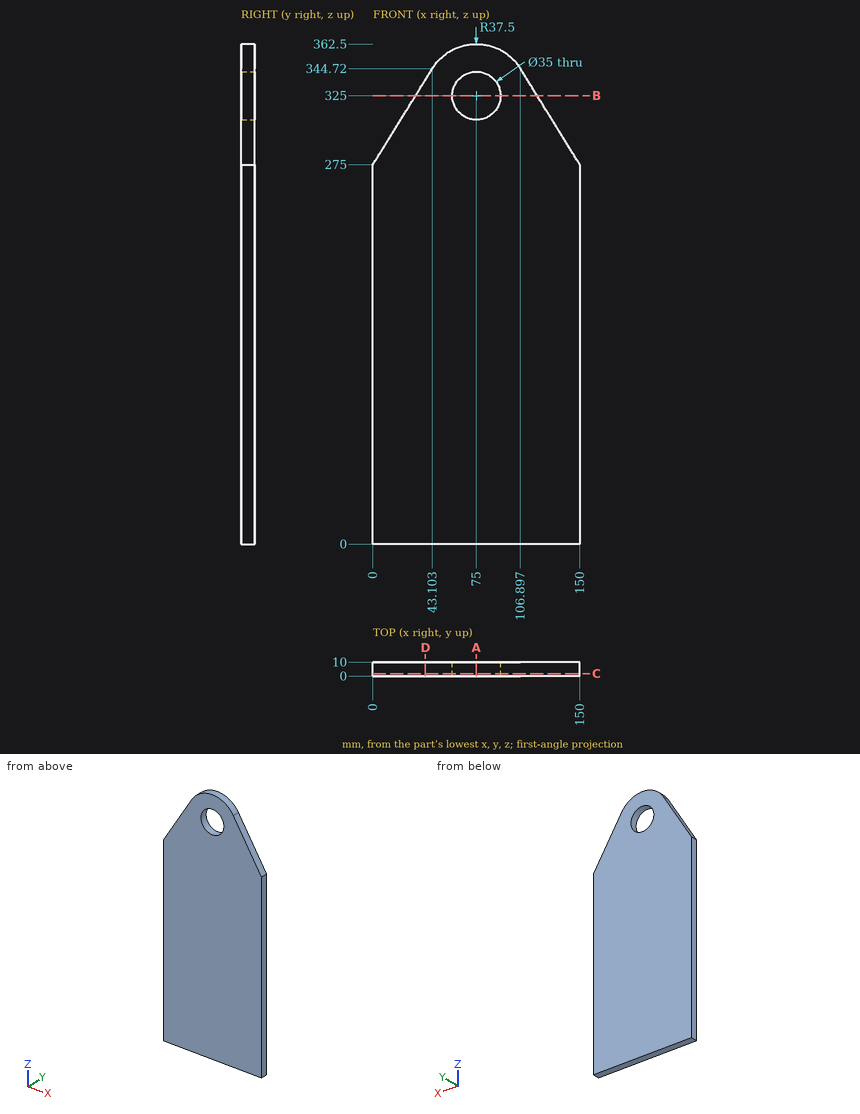
Input: dimensioned drawing with shaded views. Units: mm. Origin: part minimum x, y, z. Coordinates: 2 decimals unless noted, no trailing zeros. Order: outer loops, then holes, each group sorted by start corner. A loop starts at its lowest first (then second) coordinate and runs counter-clockwise, first axis right, second up.
1. Cut plane B-B, the plane z = 325. Return loops of the section in (x, y), plus the area to 3 significant figures.
Checked values:
outline: (30.91, 0) - (57.5, 0) - (57.5, 10) - (30.91, 10) - close; (92.5, 0) - (119.09, 0) - (119.09, 10) - (92.5, 10) - close
area: 532 mm2
2. Cut plane C-C, the plane y = 1.75. Return loops of the section in (x, z).
Checked values:
outline: (0, 0) - (150, 0) - (150, 275) - (106.9, 344.72) arc R37.5 ccw to (43.1, 344.72) - (0, 275) - close; hole circle Ø35 at (75, 325)
3. Contact query for a flat-ended pin moving along its axis: P1, Ø1, axis at x = 45.5, y = 3.5, coming from the +Z side (1 decimal). Output: stop coordinate, or through.
Checked values:
P1: stops at z = 348.8
4. Ray query, line 1 along Z through (x, y) = (75, 5); line 2 along Z through (x, y) = (63, 8.75) (1 decimal); line 3 along Z through (x, y) = (122, 6.5). Return the intervals inside material, ascending.
Checked values:
line 1: z = 0 to 307.5, 342.5 to 362.5
line 2: z = 0 to 312.3, 337.7 to 360.5
line 3: z = 0 to 320.29
5. Cut plane A-A, the plane x = 75. Return loops of the section in (y, z).
Checked values:
outline: (0, 0) - (10, 0) - (10, 307.5) - (0, 307.5) - close; (0, 342.5) - (10, 342.5) - (10, 362.5) - (0, 362.5) - close
6. Cut plane D-D, the plane x = 38. Return loops of the section in (y, z) (1 decimal).
Checked values:
outline: (0, 0) - (10, 0) - (10, 336.5) - (0, 336.5) - close
